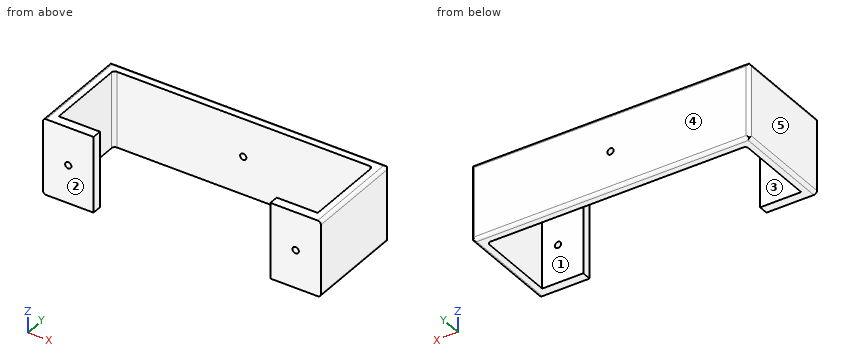
```python
from build123d import *

# Parameters (mm, degrees)
F1_DEPTH = 38.1
F2_R     = 1.5875
F3_DEPTH = 4.7625
F4_R     = 1.5875
F5_DEPTH = 4.7625
F7_DEPTH = 50.8
F9_DEPTH = 139.7


with BuildPart() as f1:
    # F0 (on Top) → F1 (new body)
    with BuildSketch(Plane.XY):
        with BuildLine():
            Line((-69.8627, -25.4), (-44.4627, -25.4))
            Line((-44.4627, -25.4), (-44.45, -20.6375))
            Line((-44.45, -20.6375), (-65.1002, -20.6375))
            Line((-65.1002, -20.6375), (-65.1002, 19.0373))
            ThreePointArc((-65.1002, 19.0373), (-64.631512, 20.168812), (-63.5, 20.6375))
            Line((-63.5, 20.6375), (63.4746, 20.6375))
            ThreePointArc((63.4746, 20.6375), (64.606112, 20.168812), (65.0748, 19.0373))
            Line((65.0748, 19.0373), (65.0748, -20.6375))
            Line((65.0748, -20.6375), (44.4373, -20.6375))
            Line((44.4373, -20.6375), (44.4373, -25.4))
            Line((44.4373, -25.4), (69.8373, -25.4))
            Line((69.8373, -25.4), (69.8373, 23.7998))
            ThreePointArc((69.8373, 23.7998), (69.368612, 24.931312), (68.2371, 25.4))
            Line((68.2371, 25.4), (-68.2625, 25.4))
            ThreePointArc((-68.2625, 25.4), (-69.394012, 24.931312), (-69.8627, 23.7998))
            Line((-69.8627, 23.7998), (-69.8627, -25.4))
        make_face()
    extrude(amount=F1_DEPTH)

    # F2 (on face) → F3 (cut)
    with BuildSketch(Plane.XZ.offset(25.4)):
        with Locations((-57.1627, 19.05)):
            Circle(F2_R)
        with Locations((57.1373, 19.05)):
            Circle(F2_R)
    extrude(amount=-F3_DEPTH, mode=Mode.SUBTRACT)

    # F4 (on face) → F5 (cut)
    with BuildSketch(Plane(origin=(0, 25.4, 0), x_dir=(-1, 0, 0), z_dir=(0, 1, 0))):
        with Locations((0, 19.05)):
            Circle(F4_R)
    extrude(amount=-F5_DEPTH, mode=Mode.SUBTRACT)

    # F6 (on face) → F7 (cut)
    with BuildSketch(Plane(origin=(0, 25.4, 0), x_dir=(-1, 0, 0), z_dir=(0, 1, 0))):
        with BuildLine():
            ThreePointArc((-69.8373, 36.4998), (-69.368612, 37.631312), (-68.2371, 38.1))
            Line((-68.2371, 38.1), (-69.8373, 38.1))
            Line((-69.8373, 38.1), (-69.8373, 36.4998))
        make_face()
        with BuildLine():
            ThreePointArc((-68.2371, 0), (-69.368612, 0.468688), (-69.8373, 1.6002))
            Line((-69.8373, 1.6002), (-69.8373, 0))
            Line((-69.8373, 0), (-68.2371, 0))
        make_face()
        with BuildLine():
            ThreePointArc((69.8627, 1.6002), (69.394012, 0.468688), (68.2625, 0))
            Line((68.2625, 0), (69.8627, 0))
            Line((69.8627, 0), (69.8627, 1.6002))
        make_face()
        with BuildLine():
            ThreePointArc((68.2625, 38.1), (69.394012, 37.631312), (69.8627, 36.4998))
            Line((69.8627, 36.4998), (69.8627, 38.1))
            Line((69.8627, 38.1), (68.2625, 38.1))
        make_face()
    extrude(amount=-F7_DEPTH, mode=Mode.SUBTRACT)

    # F8 (on face) → F9 (cut)
    with BuildSketch(Plane.YZ.offset(69.8373)):
        with BuildLine():
            ThreePointArc((23.7998, 38.1), (24.931312, 37.631312), (25.4, 36.4998))
            Line((25.4, 36.4998), (25.4, 38.1))
            Line((25.4, 38.1), (23.7998, 38.1))
        make_face()
        with BuildLine():
            ThreePointArc((25.4, 1.6002), (24.931312, 0.468688), (23.7998, 0))
            Line((23.7998, 0), (25.4, 0))
            Line((25.4, 0), (25.4, 1.6002))
        make_face()
    extrude(amount=-F9_DEPTH, mode=Mode.SUBTRACT)


solid = f1.part
```
Check sheet for the modelled part. Datum: model origin and axes. Units: mm. Face numbers are marked on the shaded views. A direction names the side the tool comes from. Coordinates: 2 decimals unless noted, no trailing zeros. Order: outer loops, then holes, each group sorted by start corner. A loop starts at its lowest first (then second) coordinate and runs counter-clockwise, first axis right, second up. Notation, with made-up numbers: (-0.5, 1.5) -> (17.5, 1.5) arc R20 ccw to (17.5, 25.5) -> close; hole circle Ø9 at (4, -28). An arc over 180 degrees is marked (long way). Write each question's results on one line, items separated by ' | '. Start each with the question number.
1) Draft check along X on the marked faces 3, 4 and 5. Enter one of: pulls with the +X half, pulls with the -X half, needs draft (parallel to the pull), parting line crosses it, or undercut.
2) Set-up check for the marked faces 1 and 2: record each of +Z, -Z, +X, -X, +Y, -Y from which the full face is reachable in a straight line by a thin tool's end or side.
3) Material ranges on line 1 along X through (y, z) = (-13, 10); line 2 along Y through (x, z) = (61, 27.5); line 3 along X through (y, z) = (22, 19), recorded low to high.
4) Section check B-B (z = 19.05). Enter the section's corners in (x, y), and give its area (3 significant figures).
5) Depth check by flat-ended pin: pin 1 (1.9 mm diameter, centred on x = -57.16, z = 19.05, fed in from -Y). Enter the tip coordinate at first touch or a pass-through.
6) Section check D-D (x = 24). Enter the section's corners in (y, z).
7) Section check A-A (y = -19). Enter the section's corners in (x, z).
8) Section check C-C (x = -47). Enter the section's corners in (y, z).
Checked values:
1) face 3: undercut | face 4: needs draft | face 5: pulls with the -X half
2) face 1: +Z, -Z | face 2: +Z, -Z, +X, -X, -Y
3) line 1: -69.86 to -65.1, 65.07 to 69.84 | line 2: -25.4 to -20.64, 20.64 to 25.4 | line 3: -69.86 to -1.59, 1.59 to 69.84
4) outline: (-69.86, -25.4) -> (-58.75, -25.4) -> (-58.75, -20.64) -> (-65.1, -20.64) -> (-65.1, 19.04) arc R1.6 cw to (-63.5, 20.64) -> (-1.59, 20.64) -> (-1.59, 25.4) -> (-68.26, 25.4) arc R1.6 ccw to (-69.86, 23.8) -> close; (-55.58, -25.4) -> (-44.46, -25.4) -> (-44.45, -20.64) -> (-55.58, -20.64) -> close; (1.59, 20.64) -> (63.47, 20.64) arc R1.6 cw to (65.07, 19.04) -> (65.07, -20.64) -> (58.72, -20.64) -> (58.72, -25.4) -> (69.84, -25.4) -> (69.84, 23.8) arc R1.6 ccw to (68.24, 25.4) -> (1.59, 25.4) -> close; (44.44, -25.4) -> (55.55, -25.4) -> (55.55, -20.64) -> (44.44, -20.64) -> close | area: 1,260 mm²
5) pin 1: y = 20.64
6) outline: (20.64, 0) -> (23.8, 0) arc R1.6 ccw to (25.4, 1.6) -> (25.4, 36.5) arc R1.6 ccw to (23.8, 38.1) -> (20.64, 38.1) -> close
7) outline: (-69.86, 1.6) arc R1.6 ccw to (-68.26, 0) -> (-65.1, 0) -> (-65.1, 38.1) -> (-68.26, 38.1) arc R1.6 ccw to (-69.86, 36.5) -> close; (65.07, 0) -> (68.24, 0) arc R1.6 ccw to (69.84, 1.6) -> (69.84, 36.5) arc R1.6 ccw to (68.24, 38.1) -> (65.07, 38.1) -> close
8) outline: (-25.4, 0) -> (-20.64, 0) -> (-20.64, 38.1) -> (-25.4, 38.1) -> close; (20.64, 0) -> (23.8, 0) arc R1.6 ccw to (25.4, 1.6) -> (25.4, 36.5) arc R1.6 ccw to (23.8, 38.1) -> (20.64, 38.1) -> close
